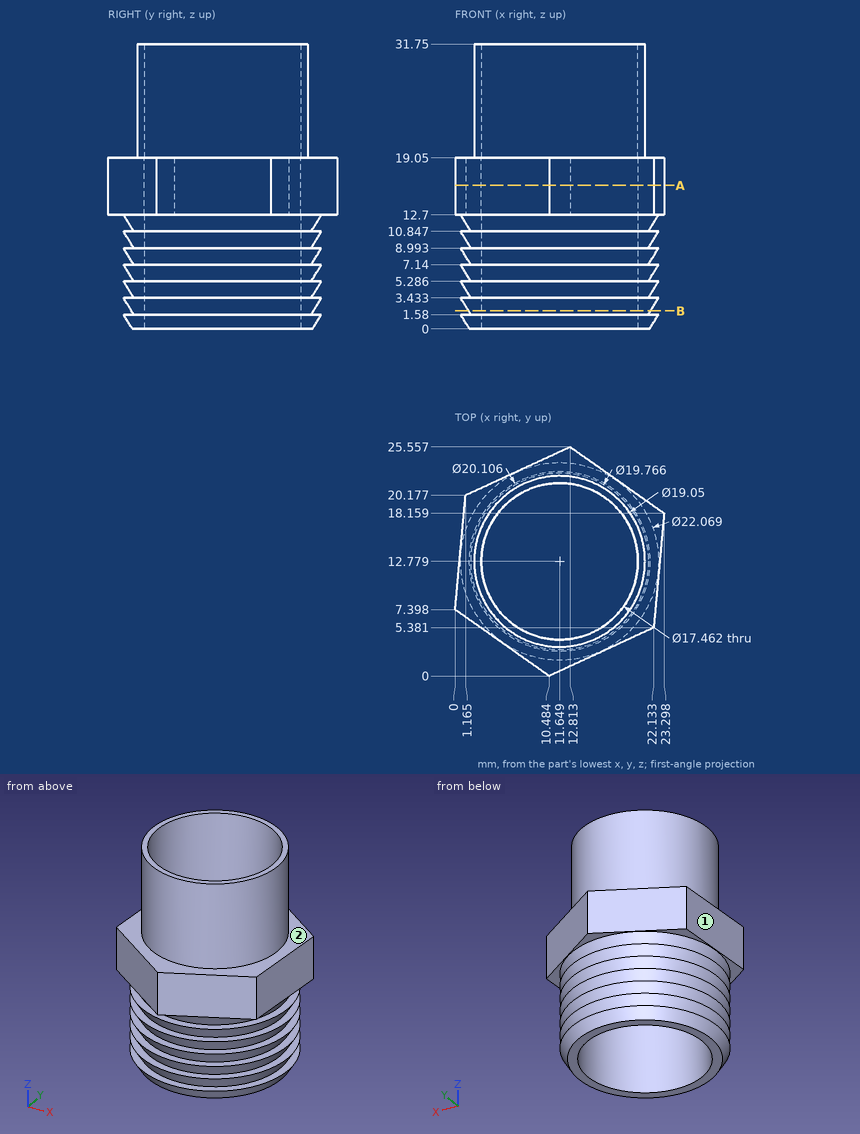
Verification items for this drawing (mm, ordinates from the low corner). A direction names the side the tool comes from. Coordinates: 2 decimals unless noted, no trailing zeros. Write each loop counter-clockwise with the first axis right and the second up, starting at its lowest first coordinate (ties: lowest second). Pieces come first, ordered by that corner, then holes. Notation, with made-up numbers: M 87.25,16.5 L 92.25,16.5 A32 ccw 92.25,49.5 Z; hole C 64,5.25 d11. An arc over 180 degrees is marked long. Answer as a JSON object with one key per item and string values.
1. Scan lines: L1, parallel to X at y = 5, z = 2 (1 decimal); L2, parallel to X at y = 14.75, z = 24 (1 decimal); L3, parallel to Z at x = 21.5, y = 19.25. Record each from-to range of solid material in increasing order.
Answers below:
{"L1": "x = 5.1 to 7.7, 15.6 to 18.2", "L2": "x = 2.3 to 3.1, 20.2 to 21", "L3": "z = 12.7 to 19.05"}
2. Section check A-A, the plane z = 16. Enter the section's corners in (x, y) (1 decimal), plus the area to 3 significant figures.
Answers below:
{"outline": "M 0,7.4 L 10.5,0 L 22.1,5.4 L 23.3,18.2 L 12.8,25.6 L 1.2,20.2 Z; hole C 11.6,12.8 d17.5", "area": "188 mm²"}
3. Go/stop test with flat-tipped pins: pin 1 Ø1 at (y, z) = (17, 27.5) entering from +X; pin 2 Ø5 at (x, z) = (15.5, 6.5) entering from -Y; pin 3 Ø5 at (y, z) = (12.5, 14) entering from +X. Record where each tip stops, or that it passes through.
Answers below:
{"pin 1": "stops at x = 20.42", "pin 2": "stops at y = 1.84", "pin 3": "stops at x = 23.01"}
4. Tool access check on the marked faces 1 and 2. Record the directions out of +Z, -Z, +X, -X, +Y, -Y that give a thin tool (end or side, any length) a straight path to the whole face; none if there is none.
Answers below:
{"face 1": "+Z, -Z, -X, +Y", "face 2": "+Z"}
5. Section check B-B, the plane z = 2. Enter the section's corners in (x, y) (1 decimal).
Answers below:
{"outline": "C 11.6,12.8 d20.3; hole C 11.6,12.8 d17.5"}
